Geometry check sheet. Reference: the model listing, model coordinates, mm. Face numbers are marked on the shaded views. A direction names the side the tool comes from. Give positions to 0.01 mm unless a question says otherwise; leave off trailing zeros. Answer as a JSON object with one key per item and string values.
from build123d import *

# Parameters (mm, degrees)
SKETCH5_W               = 180
SKETCH5_H               = 180
SKETCH5_W_2             = 160
SKETCH5_H_2             = 160
BOSS_EXTRUDE5_DEPTH     = 10
SKETCH6_W               = 10
SKETCH6_H               = 10
BOSS_EXTRUDE6_DEPTH     = 120
SKETCH7_W               = 10
SKETCH7_H               = 10
BOSS_EXTRUDE7_DEPTH     = 177.77027879
SKETCH10_R              = 2.5
SKETCH10_W              = 60
SKETCH10_H              = 5
BOSS_EXTRUDE9_DEPTH     = 5
CUT_EXTRUDE1_DEPTH      = 212.187120819
SKETCH12_W              = 160
SKETCH12_H              = 160
BOSS_EXTRUDE10_DEPTH    = 5
SKETCH14_W              = 160
SKETCH14_H              = 120
BOSS_EXTRUDE12_DEPTH    = 5
BOSS_EXTRUDE13_DEPTH    = 170.97785486
SKETCH16_W              = 160
SKETCH16_H              = 120
BOSS_EXTRUDE14_DEPTH    = 5
SKETCH17_W              = 160
SKETCH17_H              = 120
BOSS_EXTRUDE15_DEPTH    = 5
CUT_EXTRUDE2_DEPTH      = 182.934053987
CUT_EXTRUDE2_DEPTH_BACK = 125
SKETCH18_W              = 170
SKETCH18_H              = 5
BOSS_EXTRUDE16_REACH    = 234.164
SKETCH20_W              = 5
SKETCH20_H              = 5
CUT_EXTRUDE4_DEPTH      = 5
FILLET4_R               = 5
FILLET6_R               = 2.5
SKETCH9_W               = 160
SKETCH9_H               = 160
BOSS_EXTRUDE8_DEPTH     = 5


with BuildPart() as part:
    # Sketch5 → Boss-Extrude5 (new body)
    with BuildSketch(Plane(origin=(0, 0, 0), x_dir=(1, 0, 0), z_dir=(0, 1, 0))):
        Rectangle(SKETCH5_W, SKETCH5_H)
        Rectangle(SKETCH5_W_2, SKETCH5_H_2, mode=Mode.SUBTRACT)
    extrude(amount=BOSS_EXTRUDE5_DEPTH)

    # Sketch6 → Boss-Extrude6 (add)
    with BuildSketch(Plane(origin=(0, 10, 0), x_dir=(1, 0, 0), z_dir=(0, 1, 0))):
        with Locations((85, -85)):
            Rectangle(SKETCH6_W, SKETCH6_H)
        with Locations((85, 85)):
            Rectangle(SKETCH6_W, SKETCH6_H)
        with Locations((-85, 85)):
            Rectangle(SKETCH6_W, SKETCH6_H)
        with Locations((-85, -85)):
            Rectangle(SKETCH6_W, SKETCH6_H)
    extrude(amount=BOSS_EXTRUDE6_DEPTH)

    # Sketch7 → Boss-Extrude7 (add)
    with BuildSketch(Plane.XY.offset(90)):
        with Locations((85, 55)):
            Rectangle(SKETCH7_W, SKETCH7_H)
        with Locations((-85, 55)):
            Rectangle(SKETCH7_W, SKETCH7_H)
    extrude(amount=-BOSS_EXTRUDE7_DEPTH)

    # Sketch10 → Boss-Extrude9 (add)
    with BuildSketch(Plane(origin=(-80, 0, 0), x_dir=(0, 0, -1), z_dir=(1, 0, 0))):
        with Locations(Location((17.5, 57.5, 0), (0, 0, 90))):
            Circle(SKETCH10_R)
        with Locations((-20, 52.5)):
            Rectangle(SKETCH10_W, SKETCH10_H)
    boss_extrude9 = extrude(amount=BOSS_EXTRUDE9_DEPTH)

    # Sketch11 → Cut-Extrude1 (cut, symmetric)
    with BuildSketch(Plane.XY.offset(50)):
        Polygon((-75, 55), (-80, 50), (-75, 50), align=None)
    cut_extrude1 = extrude(amount=CUT_EXTRUDE1_DEPTH, both=True, mode=Mode.SUBTRACT)

    # Mirror1: Boss-Extrude9, Cut-Extrude1 across plane
    add(boss_extrude9.mirror(Plane(origin=(0, 0, 0), x_dir=(0, 0, 1), z_dir=(1, 0, 0))))
    add(cut_extrude1.mirror(Plane(origin=(0, 0, 0), x_dir=(0, 0, 1), z_dir=(1, 0, 0))), mode=Mode.SUBTRACT)

    # Sketch12 → Boss-Extrude10 (add)
    with BuildSketch(Plane.XZ):
        Rectangle(SKETCH12_W, SKETCH12_H)
    extrude(amount=-BOSS_EXTRUDE10_DEPTH)

    # Sketch14 → Boss-Extrude12 (add)
    with BuildSketch(Plane(origin=(0, 0, -90), x_dir=(-1, 0, 0), z_dir=(0, 0, -1))):
        with Locations((0, 70)):
            Rectangle(SKETCH14_W, SKETCH14_H)
    extrude(amount=-BOSS_EXTRUDE12_DEPTH)

    # Sketch15 → Boss-Extrude13 (add)
    with BuildSketch(Plane.XY.offset(90)):
        Polygon((-90, 125), (-80, 125), (-90, 115), align=None)
        Polygon((90, 115), (90, 125), (80, 125), align=None)
    extrude(amount=-BOSS_EXTRUDE13_DEPTH)

    # Sketch16 → Boss-Extrude14 (add)
    with BuildSketch(Plane(origin=(90, 0, 0), x_dir=(0, 0, -1), z_dir=(1, 0, 0))):
        with Locations((0, 70)):
            Rectangle(SKETCH16_W, SKETCH16_H)
    extrude(amount=-BOSS_EXTRUDE14_DEPTH)

    # Sketch17 → Boss-Extrude15 (add)
    with BuildSketch(Plane.ZY.offset(90)):
        with Locations((0, 70)):
            Rectangle(SKETCH17_W, SKETCH17_H)
    extrude(amount=-BOSS_EXTRUDE15_DEPTH)

    # Sketch18 → Cut-Extrude2 (cut, two sides: drawn at the far end of the back side and taken through both)
    with BuildSketch(Plane(origin=(0, 130, 0), x_dir=(1, 0, 0), z_dir=(0, 1, 0)).offset(-CUT_EXTRUDE2_DEPTH_BACK)):
        with Locations((0, -85)):
            Rectangle(SKETCH18_W, SKETCH18_H)
    extrude(amount=CUT_EXTRUDE2_DEPTH + CUT_EXTRUDE2_DEPTH_BACK, mode=Mode.SUBTRACT)

    # Sketch19 → Boss-Extrude16 (add, up to next)
    with BuildSketch(Plane(origin=(-80, 0, 0), x_dir=(0, 0, -1), z_dir=(1, 0, 0)), mode=Mode.PRIVATE) as boss_extrude16_sk1:
        Polygon((80, 125), (85, 125), (85, 120), align=None)
    boss_extrude16_tool1 = extrude(boss_extrude16_sk1.sketch, amount=BOSS_EXTRUDE16_REACH, mode=Mode.PRIVATE) - part.part
    add(boss_extrude16_tool1.solids().sort_by_distance((-80, 123.333333, -83.333333))[0])

    # Sketch20 → Cut-Extrude4 (cut)
    with BuildSketch(Plane(origin=(0, 130, 0), x_dir=(1, 0, 0), z_dir=(0, 1, 0))):
        with Locations((-82.5, 82.5)):
            Rectangle(SKETCH20_W, SKETCH20_H)
        with Locations((82.5, 82.5)):
            Rectangle(SKETCH20_W, SKETCH20_H)
    extrude(amount=-CUT_EXTRUDE4_DEPTH, mode=Mode.SUBTRACT)

    # Fillet4
    fillet4_edges = [part.edges().sort_by_distance(p)[0] for p in [
        (90, 130, 0),
        (0, 130, -90),
        (0, 0, -90),
        (-90, 130, 0),
        (90, 0, 0),
        (0, 0, 90),
        (-90, 0, 0),
        (-90, 65, -90),
        (90, 65, -90),
        (90, 65, 90),
        (-90, 65, 90),
    ]]
    fillet(fillet4_edges, radius=FILLET4_R - 0.0001)  # a hair under: the kernel refuses the full size

    # Fillet6
    fillet6_edges = [part.edges().sort_by_distance(p)[0] for p in [
        (-80, 70, 90),
        (80, 70, 90),
        (0, 10, 90),
    ]]
    fillet(fillet6_edges, radius=FILLET6_R - 0.0001)  # a hair under: the kernel refuses the full size

    # Sketch9 → Boss-Extrude8 (add)
    with BuildSketch(Plane(origin=(0, 0, 0), x_dir=(-1, 0, 0), z_dir=(0, -1, 0))):
        Rectangle(SKETCH9_W, SKETCH9_H)
    extrude(amount=-BOSS_EXTRUDE8_DEPTH)


solid = part.part
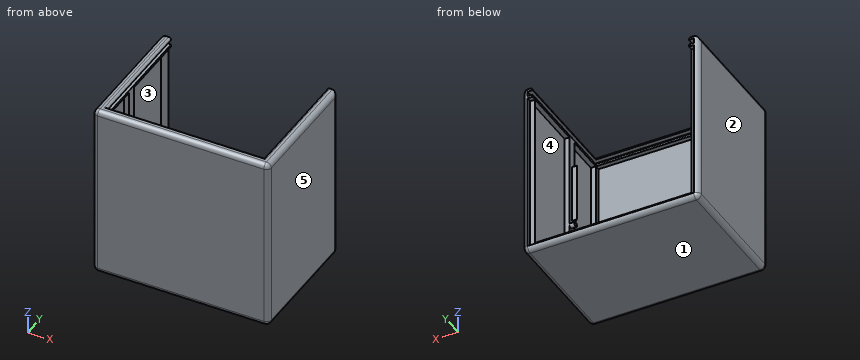
1) Tool access check on the marked faces 4 and 5. Record the directions out of +Z, -Z, +X, -X, +Y, -Y that give a thin tool (end or side, any length) a straight path to the whole face; none if there is none.
Geometry check:
{"face 4": "none", "face 5": "+Z, -Z, +X, +Y, -Y"}
2) Depth check by flat-ended pin: P1, Ø1.5, axis at x = -83, z = -23, coming from the +Y side; P2, Ø1.5, axis at x = 42, z = 17.5, coming from the +Y side; P3, Ø1.5, axis at x = -77, y = 53.5, coming from the +Z side. Enter the tip coordinate at first touch or a pass-through.
Geometry check:
{"P1": "stops at y = 125", "P2": "stops at y = 5", "P3": "stops at z = 50"}
3) Draft check along X on the marked faces 1, 2 and 3. Enter one of: pulls with the +X half, pulls with the -X half, needs draft (parallel to the pull), parting line crosses it, or undercut.
Geometry check:
{"face 1": "needs draft", "face 2": "pulls with the -X half", "face 3": "undercut"}
4) Material ranges on line 1 along X through (y, z) = (18.5, -56.5); line 2 along Z through (x, y) = (81.5, 64); line 3 along Y through (x, z) = (38.5, 34.5), recorded low to high. Write a range as from..to.
Geometry check:
{"line 1": "x = -90..-85, 85..90", "line 2": "z = -90..-80, 80..82.5, 87.5..89.79", "line 3": "y = 0..5"}
